Source: CAD feature listing. Evaluate the final solid. Frame: model axes, mm. Round coordinates to 2 decimals unless told otherwise and drop trailing zeros. Order: outer loops, then holes, each group sorted by start corner. A loop starts at its lowest first (then second) coordinate and runs counter-clockwise, first axis right, second up. Notation, with made-up numbers: (-10.75, 4.5) - (21.25, 4.5) arc R18 cw to (21.25, 34.5) - close; hole circle Ø6 at (70.25, 64). An arc over 180 degrees is marked (long way). Return JSON: item names as keys, results as strings. Group by question number.
1) Ray query, line 1 (Y direction, x = 10, z = 2.2); line 2 (X direction, y = 70, z = 3.6); line 3 (X direction, y = 18, z = 4.75). Return the intervals inside material, ascending. Write a range as from..to.
2) Section A-A, the plane x = 230. Return loops of the section in (y, z).
3) Section C-C, the plane z = 3. Give the number of separate pieces and of enclosed holes in the cut face, plus the area to 3 significant figures.
4) Mould query, pull axis Y, two halves, no side actions, for faces 1 (the flat face through (137, 80, 2)), 2 (the flat face through (133, 41, 0)), 3 (the cylindrical face through (36.9, 16.2, 2.5)), 4 (the cylindrical face through (9.879, 72.747, 2.465)). Classes: pulls with the +Y half, pulls with the -Y half, needs draft (parallel to the pull), parting line crosses it, or undercut.
5) Section B-B, the plane y = 40. Return loops of the section in (x, z).
6) Section D-D, the plane x = 182. Return loops of the section in (y, z), plus the area to 3 significant figures.
Autodesk Inventor part; units mm, degrees
ref_plane "YZ Plane" through (0, 0, 0) normal (1, 0, 0) x (0, 1, 0)
ref_plane "XZ Plane" through (0, 0, 0) normal (0, 1, 0) x (-1, 0, 0)
ref_plane "XY Plane" through (0, 0, 0) normal (0, 0, 1) x (1, 0, 0)
sketch "Sketch1" plane through (0, 0, 0) normal (0, 0, 1) x (1, 0, 0)
  line L0 (0, 0) -> (270, 0)
  line L1 (270, 0) -> (270, 80)
  line L2 (270, 80) -> (0, 80)
  line L3 (0, 80) -> (0, 0)
  circle A0 centre (40, 40) radius 24
  circle A1 centre (103.3333, 40) radius 24
  circle A2 centre (166.6667, 40) radius 24
  circle A3 centre (230, 40) radius 24
  dimension "d0" = 270
  dimension "d1" = 80
  dimension "d2" = 40
  dimension "d3" = 63.3333
  dimension "d4" = 63.3333
  dimension "d5" = 63.3333
  dimension "d6" = 48
  dimension "d7" = 48
  dimension "d8" = 48
  dimension "d9" = 48
extrude "Extrusion1" add sketch "Sketch1" along normal blind 5
sketch "Sketch2" plane through (0, 0, 5) normal (0, 0, 1) x (1, 0, 0)
  circle A0 centre (10, 70) radius 2.75
  circle A1 centre (260, 70) radius 2.75
  circle A2 centre (260, 10) radius 2.75
  circle A3 centre (10, 10) radius 2.75
  line L0 (270, 80) -> (0, 80)
  line L1 (0, 80) -> (0, 0)
  line L2 (0, 0) -> (270, 0)
  line L3 (270, 0) -> (270, 80)
  dimension "d12" = 10
  dimension "d13" = 10
  dimension "d14" = 10
  dimension "d15" = 10
  dimension "d16" = 10
  dimension "d17" = 10
  dimension "d18" = 10
  dimension "d19" = 10
  dimension "d20" = 5.5
  dimension "d21" = 5.5
  dimension "d22" = 5.5
  dimension "d23" = 5.5
hole "Hole1" at (10, 70, 5) at (260, 70, 5) at (260, 10, 5) at (10, 10, 5) direction (0, 0, -1) diameter 5.5 end through all
fillet "Fillet1" radius 2 4 edges at (0, 0, 2.5) (270, 0, 2.5) (270, 80, 2.5) (0, 80, 2.5)
equation "\"d4\" = d3"
equation "\"d5\" = d3"
equation "\"d7\" = d6"
equation "\"d8\" = d6"
equation "\"d9\" = d6"
equation "\"d13\" = d12"
equation "\"d14\" = d12"
equation "\"d15\" = d12"
equation "\"d16\" = d12"
equation "\"d17\" = d12"
equation "\"d18\" = d12"
equation "\"d19\" = d12"
equation "\"d21\" = d20"
equation "\"d22\" = d20"
equation "\"d23\" = d20"
equation "\"d24\" = d20"
properties part number "TopPlates"
Geometry check:
{
 "1": {"line 1": "0..7.25, 12.75..67.25, 72.75..80", "line 2": "0..7.25, 12.75..257.25, 262.75..270", "line 3": "0..30.41, 49.59..93.74, 112.92..157.08, 176.26..220.41, 239.59..270"},
 "2": {"outline": "(0, 0) - (16, 0) - (16, 5) - (0, 5) - close; (64, 0) - (80, 0) - (80, 5) - (64, 5) - close"},
 "3": {"separate pieces": "1", "enclosed holes": "8", "area": "14,300 mm2"},
 "4": {"face 1": "pulls with the +Y half", "face 2": "needs draft", "face 3": "undercut", "face 4": "undercut"},
 "5": {"outline": "(0, 0) - (16, 0) - (16, 5) - (0, 5) - close; (64, 0) - (79.33, 0) - (79.33, 5) - (64, 5) - close; (127.33, 0) - (142.67, 0) - (142.67, 5) - (127.33, 5) - close; (190.67, 0) - (206, 0) - (206, 5) - (190.67, 5) - close; (254, 0) - (270, 0) - (270, 5) - (254, 5) - close"},
 "6": {"outline": "(0, 0) - (21.54, 0) - (21.54, 5) - (0, 5) - close; (58.46, 0) - (80, 0) - (80, 5) - (58.46, 5) - close", "area": "215 mm2"}
}
